Autodesk Inventor part; units mm, degrees
ref_plane "Work Plane2" through (0, 0, -6.4142) normal (0, 0, -1) x (-1, 0, 0)
ref_plane "YZ Plane" through (0, 0, 0) normal (1, 0, 0) x (0, 1, 0)
ref_plane "XZ Plane" through (0, 0, 0) normal (0, 1, 0) x (-1, 0, 0)
sketch "Sketch1" plane through (0, 0, 0) normal (0, 1, 0) x (-1, 0, 0)
  line L0 (1.366, -1) -> (4.5858, -1)
  line L1 (5, 0) -> (0.5, 0)
  line L2 (4.5858, -1) -> (10, -6.4142)
  line L3 (5, 0) -> (11, -6)
  line L4 (11, -6) -> (11, -10)
  line L5 (11, -10) -> (13, -10)
  line L6 (13, -10) -> (13, -11.5)
  line L7 (13, -11.5) -> (10, -11.5)
  line L8 (10, -11.5) -> (10, -6.4142)
  line L9 (0, 0) -> (0, -4.2235)
  line L10 (10, -6.4142) -> (1.366, -6.4142)
  line L11 (1.366, -6.4142) -> (1.366, -1)
  line L12 (0.5, 0) -> (0.5, -0.5)
  line L13 (0.5, -0.5) -> (1.366, -1)
  dimension "d3" = 26
  dimension "d5" = 20
  dimension "d6" = 1
  dimension "d7" = 135
  dimension "d8" = 1
  dimension "d9" = 10
  dimension "d10" = 11.5
  dimension "d11" = 1.5
  dimension "d32" = 1
  dimension "d33" = 1
  dimension "d34" = 0.5
  dimension "d35" = 30
revolve "Revolution1" add sketch "Sketch1" angle 360 about axis through (0, 0, 0) along (0, 0, -1)
sketch "Sketch4" plane through (0, 0, -6.4142) normal (0, 0, -1) x (-1, 0, 0)
  circle A0 centre (0, 0) radius 1.366
hole "Hole2" at (0, 0, -6.4142) direction (0, 0, 1) diameter 16 depth 1.4 tip angle 118
ref_plane "Work Plane2" through (0, 0, -6.4142) normal (0, 0, -1) x (-1, 0, 0)
sketch "Sketch5" plane through (0, 0, -6.4142) normal (0, 0, -1) x (-1, 0, 0)
  circle A0 centre (0, 0) radius 10
  line L0 (0, -13.75) -> (0, -7.75) construction
  line L1 (2.25, -13.75) -> (2.25, -7.75)
  line L2 (-2.25, -7.75) -> (-2.25, -13.75)
  arc A1 (-2.25, -13.75) -> (2.25, -13.75) centre (0, -13.75) ccw
  arc A2 (2.25, -7.75) -> (-2.25, -7.75) centre (0, -7.75) ccw
  point P0 (0, -10.75)
  dimension "d37" = 4.5
  dimension "d38" = 6
extrude "Extrusion1" cut sketch "Sketch5" against normal blind 10 contours L2 A2 L1 A0 | A0 L1 A1 L2 picked at (-0.2519, -8.4905)
pattern_circular "Circular Pattern2" count 2 over 360 about axis through (0, 0, -8) along (0, 0, -1) of "Extrusion1"
properties part number "016" material "Stainless Steel, Austenitic"
Design review of the part built by this model. Coordinates are the model's own, in mm. A direction names the side the tool comes from. Give positions to 0.01 mm unless a question says otherwise; leave off trailing zeros. Write each loop counter-clockwise with the first axis right and the second up, starting at its lowest first coordinate (ties: lowest second). Pieces come first, ordered by that corner, then holes. Notation, with made-up numbers: M 50.5,81.25 L 74.5,81.25 A7 ccw 74.5,88.25 Z; hole C 85.5,11 d2. An arc over 180 degrees is marked long. Return JSON: item names as keys, results as strings. Group by question number.
Item 1: Clearance check with flat-ended pins moving along their axes: pin 1 Ø6 at (x, y) = (7.5, 5) entering from +Z; pin 2 Ø6 at (x, y) = (-6.5, 2.5) entering from -Z; pin 3 Ø1.4 at (x, y) = (1, 10.5) entering from +Z. State where each tip first meets the part, or that it passes through.
Item 2: Take a section at D-D (z = -2.5). Give the boundary of the cut face in (x, y), plus the area to 3 significant figures.
Item 3: Take a section at C-C (z = -7). Give the boundary of the cut face in (x, y), plus the area to 3 significant figures.
Item 4: Take a section at B-B (x = 0). Count the separate pieces of the cut face and the enclosed holes in it, plus the area to 3 significant figures.
Item 5: The part is to be moulded in two halves that separate along X. For faces 4 (the flat face through (8.2, -0.7, -6.414)), 5 (the flat face through (-7, -8, -11.5)), 6 (the flat face through (0, 10.4, -6.414)), 7 (the cylindrical face through (10.316, -7.91, -10.76)), say which applies: pulls with the +X half, pulls with the -X half, needs draft (parallel to the pull), parting line crosses it, or undercut.
Item 6: Wall thickness on line 1 along X through (y, z) = (-8, -4.5); line 2 along Y through (x, z) = (-6, -6.75); line 3 along Z through (x, y) = (2.75, -2): over which ranges is each line inside the solid? List them lowest first.
Item 7: Tool access review of faces 1 (the flat face through (2.25, -9, -5)), 2 (the cylindrical face through (-8, 0, -6)), 3 (the flat face through (0, -10.4, -6.414)): name each direction out of +Z, -Z, +X, -X, +Y, -Y from which nothing blocks a thin tool from reaching the whole face with its end or side.
Return value:
{
 "1": {"pin 1": "stops at z = -1.01", "pin 2": "stops at z = -6.41", "pin 3": "stops at z = -6.41"},
 "2": {"outline": "M -2.18,-7.18 A2.25 cw 2.18,-7.18 A7.5 ccw 2.18,7.18 A2.25 cw -2.18,7.18 A7.5 ccw Z; hole C 0,0 d7.63", "area": "118 mm2"},
 "3": {"outline": "C 0,0 d22; hole C 0,0 d20", "area": "66.0 mm2"},
 "4": {"separate pieces": "4", "enclosed holes": "0", "area": "36.0 mm2"},
 "5": {"face 4": "undercut", "face 5": "needs draft", "face 6": "undercut", "face 7": "parting line crosses it"},
 "6": {"line 1": "x = -5.12 to -2.25, 2.25 to 5.12", "line 2": "y = -9.22 to -8, 8 to 9.22", "line 3": "z = -2.25 to 0"},
 "7": {"face 1": "+Z, -Y", "face 2": "-Z", "face 3": "+Z, +Y, -Y"}
}
